Input: part model. Units: mm. Frame: model coordinates. A direction names the side the tool comes from. Give positions to 0.01 mm unless a question says otherwise; leave off trailing zeros. Write each loop counter-clockwise with the first axis right and the second up, starting at its lowest first coordinate (ties: lowest second). Pieces come first, ordered by that corner, then holes. Notation, with made-up numbers: (-26.5, 20) -> (3.5, 20) arc R22 ccw to (3.5, 44) -> close; hole circle Ø1 at (-6.75, 25). An arc over 180 degrees is marked (long way). Return JSON: item names as keys, results as strings. Group by question number.
Item 1: Set-up query: faces 5 (the face through (-48, 0, 9.326)), 6 (the face through (-48, 0, -9.622)), 7 (the face through (46, -1, -9.622)). Return all of +Z, -Z, +X, -X, +Y, -Y with unobstructed straight access to the full face (end or side cutting, diameter ignored); none if empty.
Item 2: Pin query (flat end, axial travel): P1, Ø3, axis at x = -14, z = -8, coming from the -Y side; P2, Ø4, axis at x = -62.5, y = -22.5, coming from the -Z side; P3, Ø1, axis at x = 2, y = 31, coming from the +Z side. Return the tip coordinate at first contact, or that it passes through.
Item 3: Mould query, pull axis Y, two halves, no side actions, for faces 1 (the face through (60.81, 1.84, -0.02)), 2 (the face through (46, -1, 9.326)), 3 (the face through (-40.705, -0.454, -0.015)), 4 (the face through (40.694, 1.024, -0.015)). Classes: released by +Y, released by -Y, zero draft, split by the parting line, or undercut.
Item 4: Section A-A, the plane y = 0. Return loops of the section in (x, z), then the cut area to 3 significant figures.
Item 5: Line query: line 1 (Y direction, x = 0, z = -2.5); line 2 (Y direction, x = 0, z = -3.75); line 3 (X direction, y = 21, z = -2.5). Output: solid intervals per line, ascending. Write a range as [from, to].
Item 6: Section B-B, the plane x = 20. Return loops of the section in (y, z), then the cut area to 3 significant figures.
Item 7: Section C-C, the plane z = -8. Return loops of the section in (x, y).
Item 8: Section D-D, the plane x = 2.5. Count the separate pieces of the cut face and the enclosed holes in it, then the cut area to 3 significant figures.
from build123d import *

# Parameters (mm, degrees)
F0_W = 20.131584
F0_H = 18.94737
F2_R = 13.652167


with BuildPart() as f1:
    # F0 (on Front) → F1 (revolve)
    with BuildSketch(Plane.XZ):
        with Locations((50.77303, -0.148026)):
            Rectangle(F0_W, F0_H)
    revolve(axis=Axis((0, 0, 10.06579), (0, 0, -1)))

    # F2 (on Front) → F3 (revolve)
    with BuildSketch(Plane.XZ):
        Circle(F2_R)
    revolve(axis=Axis((-41.595396, 0, 5.773026), (0, 0, -1)))


solid = f1.part
Answer below:
{
 "1": {"face 5": "+Z", "face 6": "-Z", "face 7": "-Z, +X"},
 "2": {"P1": "stops at y = -59.54", "P2": "stops at z = -10.37", "P3": "stops at z = 7.51"},
 "3": {"face 1": "split by the parting line", "face 2": "zero draft", "face 3": "undercut", "face 4": "undercut"},
 "4": {"outline": "circle Ø27.3 at (-83.19, 0); (-60.84, -9.62) -> (-40.71, -9.62) -> (-40.71, 9.33) -> (-60.84, 9.33) -> close; circle Ø27.3 at (0, 0); (40.71, -9.62) -> (60.84, -9.62) -> (60.84, 9.33) -> (40.71, 9.33) -> close", "area": "1,930 mm2"},
 "5": {"line 1": "y = [-60.84, -40.71], [-36.01, 36.01], [40.71, 60.84]", "line 2": "y = [-60.84, -40.71], [-35.56, 35.56], [40.71, 60.84]", "line 3": "x = [-92.45, -60.38], [-57.1, -34.87], [-22.81, 9.26], [34.87, 57.1]"},
 "6": {"outline": "(-57.46, -9.62) -> (-35.46, -9.62) -> (-35.46, 9.33) -> (-57.46, 9.33) -> close; (35.46, -9.62) -> (57.46, -9.62) -> (57.46, 9.33) -> (35.46, 9.33) -> close", "area": "834 mm2"},
 "7": {"outline": "(-31.96, -51.77) arc R60.84 ccw (long way) to (-31.96, 51.77) arc R52.66 ccw (long way) to start; hole (-54.08, -27.86) arc R60.84 cw to (-54.08, 27.86) arc R30.53 ccw to start; hole (-29.51, -28.04) arc R30.53 ccw to (-29.51, 28.04) arc R40.71 ccw to start; hole (-7.39, -40.03) arc R40.71 ccw (long way) to (-7.39, 40.03) arc R52.66 cw to start"},
 "8": {"separate pieces": "3", "enclosed holes": "0", "area": "2,260 mm2"}
}
